```python
from build123d import *

# Parameters (mm, degrees)
BOSS_EXTRUDE1_DEPTH   = 3.175
CUT_EXTRUDE5_DEPTH    = 378.611494297
F_4_CLEARANCE_HOLE1_D = 2.9464
CUT_EXTRUDE15_DEPTH   = 378.611494297


with BuildPart() as part:
    # Sketch1 → Boss-Extrude1 (new body)
    with BuildSketch(Plane.XY):
        with BuildLine():
            Line((76.2, 254), (76.2, 46.734177824))
            Line((76.2, 46.734177824), (80.01, 46.734177824))
            Line((80.01, 46.734177824), (80.01, 87.374980319))
            ThreePointArc((80.01, 87.374980319), (113.133038802, 185.356688684), (190.5, 254))
            Line((190.5, 254), (266.7, 254))
            Line((266.7, 254), (266.7, 203.2))
            Line((266.7, 203.2), (279.4, 203.2))
            Line((279.4, 203.2), (279.4, 184.15))
            Line((279.4, 184.15), (266.7, 184.15))
            Line((266.7, 184.15), (266.7, 120.65))
            Line((266.7, 120.65), (279.4, 120.65))
            Line((279.4, 120.65), (279.4, 101.6))
            Line((279.4, 101.6), (266.7, 101.6))
            Line((266.7, 101.6), (266.7, 38.1))
            Line((266.7, 38.1), (279.4, 38.1))
            Line((279.4, 38.1), (279.4, 19.05))
            Line((279.4, 19.05), (266.7, 19.05))
            Line((266.7, 19.05), (266.7, 0))
            Line((266.7, 0), (0, 0))
            Line((0, 0), (0, 19.05))
            Line((0, 19.05), (-12.7, 19.05))
            Line((-12.7, 19.05), (-12.7, 38.1))
            Line((-12.7, 38.1), (0, 38.1))
            Line((0, 38.1), (0, 101.6))
            Line((0, 101.6), (-12.7, 101.6))
            Line((-12.7, 101.6), (-12.7, 120.65))
            Line((-12.7, 120.65), (0, 120.65))
            Line((0, 120.65), (0, 184.15))
            Line((0, 184.15), (-12.7, 184.15))
            Line((-12.7, 184.15), (-12.7, 203.2))
            Line((-12.7, 203.2), (0, 203.2))
            Line((0, 203.2), (0, 254))
            Line((0, 254), (76.2, 254))
        make_face()
    extrude(amount=BOSS_EXTRUDE1_DEPTH)

    # Sketch10 → Cut-Extrude5 (cut, through all)
    with BuildSketch(Plane.XY.offset(3.175)):
        Polygon((12.7, 12.7), (12.7, 241.3), (37.714116927, 236.889336287), (37.714116927, 17.110663713), align=None)
    extrude(amount=-CUT_EXTRUDE5_DEPTH, mode=Mode.SUBTRACT)

    # #4 Clearance Hole1 (through all)
    with Locations(Plane.XY.offset(3.175)):
        with Locations((-6.35, 193.675), (-6.35, 111.125), (-6.35, 28.575), (273.05, 193.675), (273.05, 111.125), (273.05, 28.575), (47.874116927, 235.097854163), (47.874116927, 18.902145837)):
            Hole(F_4_CLEARANCE_HOLE1_D / 2)

    # Sketch21 → Cut-Extrude15 (cut, through all)
    with BuildSketch(Plane.XY.offset(3.175)):
        Polygon((158.526152675, 202.69099682), (157.974819711, 199.564232204), (176.735407405, 196.256234419), (177.286740369, 199.382999035), align=None)
        Polygon((239.522435721, 163.996596363), (240.073768685, 160.869831747), (258.83435638, 164.177829531), (258.283023416, 167.304594147), align=None)
        Polygon((120.16783778, 145.92910773), (119.067835825, 142.950749004), (136.937988179, 136.350737274), (138.037990134, 139.329096), align=None)
        Polygon((165.43889041, 129.209078013), (164.338888455, 126.230719288), (182.20904081, 119.630707557), (183.309042765, 122.609066283), align=None)
        Polygon((236.492169338, 87.476937109), (237.043502302, 84.350172493), (255.804089997, 87.658170277), (255.252757033, 90.784934893), align=None)
        Polygon((187.714641331, 78.876142869), (188.265974296, 75.749378253), (207.02656199, 79.057376038), (206.475229026, 82.184140653), align=None)
        Polygon((228.266083104, 162.011797692), (228.817416068, 158.885033076), (210.056828373, 155.577035291), (209.505495409, 158.703799907), align=None)
        Polygon((106.695880011, 35.721968707), (107.247212975, 32.595204091), (126.00780067, 35.903201876), (125.456467706, 39.029966491), align=None)
        Polygon((157.974819711, 44.763829318), (158.526152675, 41.637064702), (177.286740369, 44.945062487), (176.735407405, 48.071827103), align=None)
    extrude(amount=-CUT_EXTRUDE15_DEPTH, mode=Mode.SUBTRACT)


solid = part.part
```
The listing builds one solid part. Answer for the finished solid, in the listing's coordinates (mm). A direction names the side the tool comes from. Coordinates: 2 decimals unless noted, no trailing zeros. Loops run counter-clockwise (first coordinate to the right, second up) from the corner with the lowest first, then second, coordinate; pieces in that order, holes last. Notation, with made-up numbers: (35, -10.5) - (88, -10.5) arc R19 cw to (88, 18.5) - close; hole circle Ø10 at (24.25, 83). An arc over 180 degrees is marked (long way). Write item = value, one per line.
1) Determine the mould class of faces 3 (the face through (129.228, 142.583, 1.61)), 4 (the face through (112.328, 184.133, 1.565)), 5 (the face through (135, 129, 3.175)) for opening direction Y: pulls with the +Y half, pulls with the -Y half, needs draft (parallel to the pull), parting line crosses it, or undercut.
Responses:
face_3 = undercut
face_4 = pulls with the +Y half
face_5 = needs draft
2) Each of these flat-tipped pins is pushed along its axis until it touches: P1, Ø1.6, axis at y = 6.5, z = 1, coming from the +X side; P2, Ø1.6, axis at x = 275, z = 1, coming from the -Y side; P3, Ø1, axis at y = 224.5, z = 2, coming from the -X side; P4, Ø4, axis at x = 234, y = 95.5, coming from the -Z side. Where does it stop, or does it pass through?
Responses:
P1 = 266.7
P2 = 19.05
P3 = 0
P4 = 0
3) Find the intervals of material crossed by line 1 along Y through (x, z) = (-6.35, 1.45); line 2 along X through (y, z) = (196, 2.5); line 3 along X through (y, z) = (57.5, 2.95), in increasing order.
Responses:
line_1 = 19.05 to 27.1, 30.05 to 38.1, 101.6 to 109.65, 112.6 to 120.65, 184.15 to 192.2, 195.15 to 203.2
line_2 = -12.7 to 12.7, 37.71 to 76.2, 120.7 to 279.4
line_3 = 0 to 12.7, 37.71 to 76.2, 80.01 to 266.7
4) Section B-B (z = 1.2) is taken. Count the separate pieces of the cut face and the enclosed holes in it, plus the area to 3 significant figures.
Responses:
separate_pieces = 1
enclosed_holes = 18
area = 56,600 mm^2
5) Which of the six approach directions +Z, -Z, +X, -X, +Y, -Y give full straight-line access (tool end or side, diameter ignored) to faces 1 (the face through (135, 129, 0)), 2 (the face through (127.878, 139.697, 1.61))?
Responses:
face_1 = -Z, +X, -X, +Y, -Y
face_2 = +Z, -Z
6) Section A-A (x = 113.5) is taken. Determine the outline of the cut face in (y, z) (3 decimals), plus the area to 3 significant figures.
Responses:
outline = (0, 0) - (33.698, 0) - (33.698, 3.175) - (0, 3.175) - close; (36.922, 0) - (185.908, 0) - (185.908, 3.175) - (36.922, 3.175) - close
area = 580 mm^2
